```python
from build123d import *

# Parameters (mm, degrees)
SKETCH1_R           = 1.651
BOSS_EXTRUDE1_DEPTH = 3.175
CUT_EXTRUDE2_DEPTH  = 6.35
SKETCH7_R           = 4.9784
SKETCH7_R_2         = 1.5875
CUT_EXTRUDE3_DEPTH  = 124.96234811
FILLET1_R           = 6.35
SKETCH8_W           = 50.8
SKETCH8_H           = 12.7
CUT_EXTRUDE4_DEPTH  = 50.8
CUT_EXTRUDE5_DEPTH  = 19.304
FILLET6_R           = 6.35
FILLET7_R           = 6.35
FILLET8_R           = 19.05
BOSS_EXTRUDE2_DEPTH = 3.175
FILLET9_R           = 24.13
SKETCH13_W          = 41.667851519
SKETCH13_H          = 9.459584315
SKETCH13_W_2        = 28.967851519
SKETCH13_H_2        = 8.468235606
BOSS_EXTRUDE3_DEPTH = 3.175
BOSS_EXTRUDE4_DEPTH = 3.175
CUT_EXTRUDE9_DEPTH  = 119.214793194
SKETCH20_R          = 1.27
CUT_EXTRUDE10_DEPTH = 3.81
SKETCH21_R          = 1.27
CUT_EXTRUDE11_DEPTH = 6.35
SKETCH22_R          = 1.27
CUT_EXTRUDE12_DEPTH = 6.35
BOSS_EXTRUDE5_DEPTH = 3.175
SKETCH24_R          = 4.09575
CUT_EXTRUDE13_DEPTH = 3.175


with BuildPart() as part:
    # Sketch1 → Boss-Extrude1 (new body)
    with BuildSketch(Plane.XY):
        with BuildLine():
            Line((0, 0), (107.95, 0))
            Line((107.95, 0), (100.9362606, 26.175631792))
            Line((100.9362606, 26.175631792), (100.868755024, 26.427566033))
            ThreePointArc((100.868755024, 26.427566033), (110.348359368, 43.438223217), (95.367453293, 55.88))
            Line((95.367453293, 55.88), (0, 38.1))
            Line((0, 38.1), (0, 25.4))
            Line((0, 25.4), (-7.62, 25.4))
            Line((-7.62, 25.4), (-7.62, 12.7))
            Line((-7.62, 12.7), (0, 12.7))
            Line((0, 12.7), (0, 0))
        make_face()
        with Locations((25.817011896, 25.817011896)):
            Circle(SKETCH1_R, mode=Mode.SUBTRACT)
        with Locations((25.817011896, 12.282988104)):
            Circle(SKETCH1_R, mode=Mode.SUBTRACT)
        with Locations((12.282988104, 12.282988104)):
            Circle(SKETCH1_R, mode=Mode.SUBTRACT)
        with Locations((12.282988104, 25.817011896)):
            Circle(SKETCH1_R, mode=Mode.SUBTRACT)
    extrude(amount=BOSS_EXTRUDE1_DEPTH)

    # Sketch6 → Cut-Extrude2 (cut)
    with BuildSketch(Plane.XY.offset(3.175)):
        with BuildLine():
            Line((50.8, 0), (76.2, 0))
            ThreePointArc((76.2, 0), (63.5, 12.7), (50.8, 0))
        make_face()
    extrude(amount=-CUT_EXTRUDE2_DEPTH, mode=Mode.SUBTRACT)

    # Sketch7 → Cut-Extrude3 (cut, through all)
    with BuildSketch(Plane.XY.offset(3.175)):
        with Locations((19.05, 19.05)):
            Circle(SKETCH7_R)
        with Locations((80.766582748, 12.282988104)):
            Circle(SKETCH7_R_2)
        with Locations((94.299702748, 12.282988104)):
            Circle(SKETCH7_R_2)
        with Locations((80.766582748, 25.817011896)):
            Circle(SKETCH7_R_2)
        with Locations((94.299702748, 25.817011896)):
            Circle(SKETCH7_R_2)
    extrude(amount=-CUT_EXTRUDE3_DEPTH, mode=Mode.SUBTRACT)

    # Fillet1
    fillet1_edges = [part.edges().sort_by_distance(p)[0] for p in [
        (100.868755024, 26.427566033, 1.5875),
    ]]
    fillet(fillet1_edges, radius=FILLET1_R)

    # Sketch8 → Cut-Extrude4 (cut)
    with BuildSketch(Plane.XY.offset(3.175)):
        with Locations((25.4, 44.45)):
            Rectangle(SKETCH8_W, SKETCH8_H)
    extrude(amount=-CUT_EXTRUDE4_DEPTH, mode=Mode.SUBTRACT)

    # Sketch9 → Cut-Extrude5 (cut)
    with BuildSketch(Plane.XY.offset(3.175)):
        Polygon((50.8, 47.57098794), (50.8, 40.64), (57.15, 40.64), (57.15, 48.754861432), align=None)
    extrude(amount=-CUT_EXTRUDE5_DEPTH, mode=Mode.SUBTRACT)

    # Fillet6
    fillet6_edges = [part.edges().sort_by_distance(p)[0] for p in [
        (57.15, 40.64, 1.5875),
    ]]
    fillet(fillet6_edges, radius=FILLET6_R - 0.0001)  # a hair under: the kernel refuses the full size

    # Fillet7
    fillet7_edges = [part.edges().sort_by_distance(p)[0] for p in [
        (57.15, 48.754861432, 1.5875),
    ]]
    fillet(fillet7_edges, radius=FILLET7_R)

    # Fillet8
    fillet8_edges = [part.edges().sort_by_distance(p)[0] for p in [
        (50.8, 0, 1.5875),
    ]]
    fillet(fillet8_edges, radius=FILLET8_R)

    # Sketch12 → Boss-Extrude2 (add)
    with BuildSketch(Plane.XY.offset(3.175)):
        with BuildLine():
            Line((50.8, 40.64), (85.027112904, 40.64))
            Line((85.027112904, 40.64), (95.367453293, 55.88))
            add(Edge.make_bspline(
                [(50.8, 40.64), (70.777788932, 52.178803671), (78.594281742, 111.543427795), (95.367453293, 55.88)],
                knots=[0, 0, 0, 0, 1, 1, 1, 1], degree=3))
        make_face()
    extrude(amount=-BOSS_EXTRUDE2_DEPTH)

    # Fillet9
    fillet9_edges = [part.edges().sort_by_distance(p)[0] for p in [
        (95.367453293, 55.88, 1.5875),
    ]]
    fillet(fillet9_edges, radius=FILLET9_R)

    # Sketch13 → Boss-Extrude3 (add)
    with BuildSketch(Plane(origin=(0, 0, 0), x_dir=(-1, 0, 0), z_dir=(0, 0, -1))):
        with Locations((-29.966074241, 33.370207843)):
            Rectangle(SKETCH13_W, SKETCH13_H)
        with Locations((-23.616074241, 4.234117803)):
            Rectangle(SKETCH13_W_2, SKETCH13_H_2)
    extrude(amount=BOSS_EXTRUDE3_DEPTH)

    # Sketch18 → Boss-Extrude4 (add)
    with BuildSketch(Plane.XY.offset(3.175)):
        Polygon((0, 0), (7.62, 0), (7.62, 38.1), (0, 38.1), (0, 25.4), (-7.62, 25.4), (-7.62, 12.7), (0, 12.7), align=None)
    extrude(amount=BOSS_EXTRUDE4_DEPTH)

    # Sketch19 → Cut-Extrude9 (cut, through all)
    with BuildSketch(Plane(origin=(0, 38.1, 0), x_dir=(1, 0, 0), z_dir=(0, 1, 0))):
        Polygon((9.132148481, 0), (12.307148481, 3.175), (9.132148481, 3.175), align=None)
    extrude(amount=-CUT_EXTRUDE9_DEPTH, mode=Mode.SUBTRACT)

    # Sketch20 → Cut-Extrude10 (cut)
    with BuildSketch(Plane(origin=(18.309536053, 38.1, -53.667404751), x_dir=(0.9999106684671757, 0, -0.013366191885729645), z_dir=(0, 1, 0))):
        with Locations(Location((-1.073815344, -53.657845266, 0), (0, 0, 269.234150812))):
            Circle(SKETCH20_R)
        with Locations(Location((20.514255988, -53.946421349, 0), (0, 0, 269.234150812))):
            Circle(SKETCH20_R)
    extrude(amount=-CUT_EXTRUDE10_DEPTH, mode=Mode.SUBTRACT)

    # Sketch21 → Cut-Extrude11 (cut)
    with BuildSketch(Plane(origin=(0, -69.83828079, -53.667404751), x_dir=(0, 0.0318826428364363, 0.9994916193174229), z_dir=(-1, 0, 0))):
        with Locations(Location((59.242590915, 74.337262051, 0), (0, 0, 268.172949503))):
            Circle(SKETCH21_R)
        with Locations(Location((60.052410043, 99.724349182, 0), (0, 0, 268.172949503))):
            Circle(SKETCH21_R)
    extrude(amount=-CUT_EXTRUDE11_DEPTH, mode=Mode.SUBTRACT)

    # Sketch22 → Cut-Extrude12 (cut)
    with BuildSketch(Plane(origin=(18.309536053, 0, -53.667404751), x_dir=(0.9999106684671757, 0, -0.013366191885729645), z_dir=(0, -1, 0))):
        with Locations(Location((-5.686004931, 53.481882136, 0), (0, 0, 270.765849188))):
            Circle(SKETCH22_R)
        with Locations(Location((13.362293303, 53.736508092, 0), (0, 0, 270.765849188))):
            Circle(SKETCH22_R)
        with Locations((67.946889168, 56.879377031)):
            Circle(SKETCH22_R)
        with Locations((79.375868109, 57.032152605)):
            Circle(SKETCH22_R)
    extrude(amount=-CUT_EXTRUDE12_DEPTH, mode=Mode.SUBTRACT)

    # Sketch23 → Boss-Extrude5 (add)
    with BuildSketch(Plane.XY.offset(3.175)):
        Polygon((76.2, 0), (76.2, 8.89), (105.567931679, 8.89), (107.95, 0), align=None)
    extrude(amount=BOSS_EXTRUDE5_DEPTH)

    # Sketch24 → Cut-Extrude13 (cut)
    with BuildSketch(Plane(origin=(18.309536053, -69.83828079, 3.175), x_dir=(0.9998147472374107, 0.019247628596600598, 0), z_dir=(0, 0, 1))):
        with Locations(Location((73.496743516, 119.633445733, 0), (0, 0, 358.897124011))):
            Circle(SKETCH24_R)
    extrude(amount=-CUT_EXTRUDE13_DEPTH, mode=Mode.SUBTRACT)


solid = part.part
```
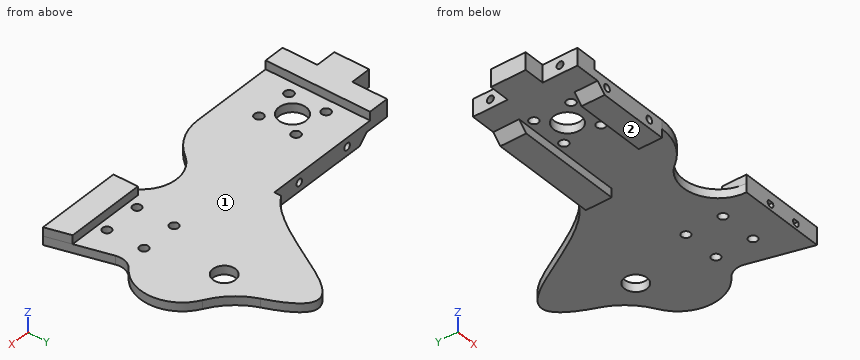
For this review, take the finished solid that the model builds, in its own axes (mm). Face numbers are marked on the shaded views. Give positions to 0.01 mm unless a question says otherwise; leave off trailing zeros. Write each loop counter-clockwise with the first axis right and the second up, starting at its lowest first coordinate (ties: lowest second). Pieces come first, ordered by that corner, then holes. Notation, with made-up numbers: M 20.25,-8 L 58.25,-8 A37 cw 58.25,28 Z; hole C 33.5,71.25 d7. An arc over 180 degrees is marked long. Answer as CSV lines item,"result".
1. Consider section C-C, the plane y = 36. Write out the cut boundary in (x, z) (3 decimals), then the cut area to 3 significant figures.
Findings:
outline,"M 0,0 L 9.132,0 L 12.307,-3.175 L 50.8,-3.175 L 50.8,0 L 109.884,0 L 109.884,3.175 L 7.62,3.175 L 7.62,6.35 L 0,6.35 Z; hole C 17.953,0 d2.54; hole C 39.543,0 d2.54"
area,"490 mm2"
2. Wall thickness on line 1 (Y direction, x = 5, z = 3); line 2 (X direction, y = 13, z = 3); line 3 (Z direction, x = 73.5, y = 46.5) (3 decimals): over which ranges is each line inside the solid? List them lowest first.
Findings:
line 1,"y = 0 to 5.09, 7.61 to 30.49, 33.01 to 38.1"
line 2,"x = -7.62 to 10.8, 13.77 to 24.33, 27.3 to 79.35, 82.18 to 92.88, 95.72 to 104.47"
line 3,"z = 0 to 3.175"
3. Draft analysis for pull direction X (two halves, no side actions). For the marked faces 1 and 2, state which applies: +X half, -X half, draft (parallel to the pull), parting line (faces both ways), or undercut.
Findings:
face 1,"undercut"
face 2,"draft"
4. Consider section B-B, the plane x = 35.5. Write out the cut boundary in (y, z) (3 decimals), then the cut area to 3 significant figures.
Findings:
outline,"M 0,-3.175 L 8.468,-3.175 L 8.468,0 L 28.64,0 L 28.64,-3.175 L 38.1,-3.175 L 38.1,3.175 L 0,3.175 Z"
area,"178 mm2"
5. Consider section A-A, the plane y = 19.05. Write out the cut boundary in (x, z) (3 decimals).
Findings:
outline,"M -7.62,0 L 14.072,0 L 14.072,3.175 L 7.62,3.175 L 7.62,6.35 L -7.62,6.35 Z; M 24.028,0 L 102.846,0 L 102.846,3.175 L 24.028,3.175 Z"
6. For pin 1 (4 mm diameter, centred on x = 72.5, y = 15, fed in from -Z); pin 2 (5 mm diameter, centred on y = 22, z = 1.5, fed in from +X) (3 decimals); pin 3 (1.5 mm diameter, centred on x = 96, z = -1.5, fed in from +Y); pin 4 (1.3 mm diameter, centred on x = 40, z = 0, fed in from +Y), all flat-tipped, find the tip position at first contact; note any pin that passes through.
Findings:
pin 1,"stops at z = 0"
pin 2,"stops at x = 102.725"
pin 3,"passes through"
pin 4,"stops at y = 34.29"
